from build123d import *

# Parameters (mm, degrees)
BOSS_EXTRUDE1_DEPTH = 19.05


with BuildPart() as part:
    # Sketch1 → Boss-Extrude1 (new body)
    with BuildSketch(Plane.XY):
        with BuildLine():
            Line((276.225, 0), (257.175, 0))
            Line((257.175, 0), (257.175, 76.2))
            Line((257.175, 76.2), (257.175, 165.1))
            Line((257.175, 165.1), (257.175, 254))
            ThreePointArc((257.175, 254), (248.194743879, 257.719743879), (244.475, 266.7))
            Line((244.475, 266.7), (231.775, 266.7))
            ThreePointArc((231.775, 266.7), (219.598293765, 286.273293765), (200.025, 298.45))
            Line((200.025, 298.45), (200.025, 311.15))
            ThreePointArc((200.025, 311.15), (191.044743879, 314.869743879), (187.325, 323.85))
            Line((187.325, 323.85), (-187.325, 323.85))
            ThreePointArc((-187.325, 323.85), (-191.044743879, 314.869743879), (-200.025, 311.15))
            Line((-200.025, 311.15), (-200.025, 298.45))
            ThreePointArc((-200.025, 298.45), (-219.598293765, 286.273293765), (-231.775, 266.7))
            Line((-231.775, 266.7), (-244.475, 266.7))
            ThreePointArc((-244.475, 266.7), (-248.194743879, 257.719743879), (-257.175, 254))
            Line((-257.175, 254), (-257.175, 165.1))
            Line((-257.175, 165.1), (-257.175, 76.2))
            Line((-257.175, 76.2), (-257.175, 0))
            Line((-257.175, 0), (-276.225, 0))
            Line((-276.225, 0), (-276.225, 330.2))
            ThreePointArc((-276.225, 330.2), (-272.505256121, 339.180256121), (-263.525, 342.9))
            Line((-263.525, 342.9), (263.525, 342.9))
            ThreePointArc((263.525, 342.9), (272.505256121, 339.180256121), (276.225, 330.2))
            Line((276.225, 330.2), (276.225, 0))
        make_face()
    extrude(amount=BOSS_EXTRUDE1_DEPTH)


solid = part.part
Can you work these out from the model? Positions are in its coordinate system, mm. A direction names the side the tool comes from. Give positions to 0.01 mm unless a question says otherwise; leave off trailing zeros. Loops run counter-clockwise (first coordinate to the right, second up) from the corner with the lowest first, then second, coordinate; pieces in that order, holes last. Notation, with made-up numbers: M 89.25,-28 L 93.25,-28 A19 cw 93.25,-12 Z; hole C 22,28.5 d6. An arc over 180 degrees is marked long. One line per item, written item: value. Start each with the question number.
1) If we section it at D-D, the plane y = 280: Write out the boundary of the cut face in (x, z) (3 decimals), and give its area (3 significant figures).
2) I'm going to push flat-ended pins straight in: pin 1 (6.5 mm diameter, centred on x = 236, z = 7, fed in from -Y); pin 2 (2 mm diameter, centred on x = -198.5, z = 6, fed in from -Y); pin 3 (9.5 mm diameter, centred on x = -35.5, z = 11, fed in from -Y). Where does each tip first touch, or does it pass through?
3) If we section it at C-C, the plane x = 142: Write out the boundary of the cut face in (y, z).
4) If I drill on line 1 (X direction, y = 311, z = 10.25) (3 decimals); line 2 (X direction, y = 206.5, z = 6) (3 decimals); line 3 (Y direction, x = -186.5, z = 4.5), over which ranges is the centre line in solid material (lowest first)? Write a range as [from, to].
5) On a 3-axis mill with a long thin cutter (end or side, diameter ignored), from which of +Z, -Z, +X, -X, +Y, -Y can I reach the whole of each face in a straight line? I mean faces 1 (the face through (276.225, 167, 9)), 2 (the face through (3, 323.85, 9)). Say none if no direction works.
6) If we section it at A-A, the plane y = 241.5: Write out the boundary of the cut face in (x, z) (3 decimals), and give its area (3 significant figures).
7) If we section it at B-B, the plane z = 4.25: Write out the boundary of the cut face in (x, y) (3 decimals), and give its area (3 significant figures).
Completed:
1. outline: M -276.225,0 L -224.928,0 L -224.928,19.05 L -276.225,19.05 Z; M 224.928,0 L 276.225,0 L 276.225,19.05 L 224.928,19.05 Z
1. area: 1,950 mm^2
2. pin 1: stops at y = 266.7
2. pin 2: stops at y = 311.16
2. pin 3: stops at y = 323.85
3. outline: M 323.85,0 L 342.9,0 L 342.9,19.05 L 323.85,19.05 Z
4. line 1: x = [-276.225, -200.025], [200.025, 276.225]
4. line 2: x = [-276.225, -257.175], [257.175, 276.225]
4. line 3: y = [323.85, 342.9]
5. face 1: +Z, -Z, +X, +Y, -Y
5. face 2: +Z, -Z, -Y
6. outline: M -276.225,0 L -257.175,0 L -257.175,19.05 L -276.225,19.05 Z; M 257.175,0 L 276.225,0 L 276.225,19.05 L 257.175,19.05 Z
6. area: 726 mm^2
7. outline: M -276.225,0 L -257.175,0 L -257.175,254 A12.7 ccw -244.475,266.7 L -231.775,266.7 A50.8 cw -200.025,298.45 L -200.025,311.15 A12.7 ccw -187.325,323.85 L 187.325,323.85 A12.7 ccw 200.025,311.15 L 200.025,298.45 A50.8 cw 231.775,266.7 L 244.475,266.7 A12.7 ccw 257.175,254 L 257.175,0 L 276.225,0 L 276.225,330.2 A12.7 ccw 263.525,342.9 L -263.525,342.9 A12.7 ccw -276.225,330.2 Z
7. area: 28,500 mm^2
